Geometry check sheet. Reference: the model listing, model coordinates, mm. A direction names the side the tool comes from. Give positions to 0.01 mm unless a question says otherwise; leave off trailing zeros. Order: outer loops, then holes, each group sorted by start corner. A loop starts at its lowest first (then second) coordinate and runs counter-clockwise, first axis right, second up. Notation, with made-up numbers: (68.25, -13) - (77.25, -13) arc R19 ccw to (77.25, 16) - close; hole circle Ø1 at (48.5, 45.5). An arc over 180 degrees is marked (long way). Put each result on its own line as item: value. Start each with the question number.
```python
from build123d import *

# Parameters (mm, degrees)
SKETCH2_R             = 22.5
BOSS_EXTRUDE2_DEPTH   = 45
M4_TAPPED_HOLE2_D     = 3.3
M4_TAPPED_HOLE2_DEPTH = 10.1
M4_TAPPED_HOLE2_TIP   = 0.991420021
SKETCH6_R             = 12
BOSS_EXTRUDE3_DEPTH   = 2
SKETCH7_R             = 5
BOSS_EXTRUDE4_DEPTH   = 25
CUT_EXTRUDE1_START    = -20
CUT_EXTRUDE1_DEPTH    = 20
SKETCH9_R             = 21
BOSS_EXTRUDE5_DEPTH   = 70
SKETCH10_R            = 18.5
BOSS_EXTRUDE6_DEPTH   = 3
SKETCH11_R            = 19.5
BOSS_EXTRUDE7_DEPTH   = 1
SKETCH12_R            = 18.5
BOSS_EXTRUDE8_DEPTH   = 7
SKETCH13_W            = 5
SKETCH13_H            = 1.5
BOSS_EXTRUDE9_DEPTH   = 7
SKETCH14_R            = 1.25
CUT_EXTRUDE2_DEPTH    = 100.047968177
FILLET1_R             = 1
FILLET2_R             = 0.5
FILLET3_R             = 0.5


with BuildPart() as part:
    # Sketch2 → Boss-Extrude2 (new body)
    with BuildSketch(Plane.XY):
        with Locations(Location((0, 0, 0), (0, 0, 180))):
            Circle(SKETCH2_R)
    extrude(amount=BOSS_EXTRUDE2_DEPTH)

    # M4 Tapped Hole2
    with Locations(Plane(origin=(0, 17, 45), x_dir=(1, 0, 0), z_dir=(0, 0, 1))):
        with Locations((0, 0), (17, -17), (0, -34), (-17, -17)):
            Hole(M4_TAPPED_HOLE2_D / 2, depth=M4_TAPPED_HOLE2_DEPTH)
            with Locations((0, 0, -(M4_TAPPED_HOLE2_DEPTH + M4_TAPPED_HOLE2_TIP / 2))):  # 118° drill point
                Cone(0, M4_TAPPED_HOLE2_D / 2, M4_TAPPED_HOLE2_TIP, mode=Mode.SUBTRACT)

    # Sketch6 → Boss-Extrude3 (add)
    with BuildSketch(Plane.XY.offset(45)):
        Circle(SKETCH6_R)
    extrude(amount=BOSS_EXTRUDE3_DEPTH)

    # Sketch7 → Boss-Extrude4 (add)
    with BuildSketch(Plane.XY.offset(47)):
        Circle(SKETCH7_R)
    extrude(amount=BOSS_EXTRUDE4_DEPTH)

    # Sketch8 → Cut-Extrude1 (cut)
    with BuildSketch(Plane.XY.offset(72).offset(CUT_EXTRUDE1_START)):
        with BuildLine():
            Line((-3.570714214, 3.5), (3.570714214, 3.5))
            ThreePointArc((3.570714214, 3.5), (0, 5), (-3.570714214, 3.5))
        make_face()
    extrude(amount=CUT_EXTRUDE1_DEPTH, mode=Mode.SUBTRACT)

    # Sketch9 → Boss-Extrude5 (add)
    with BuildSketch(Plane(origin=(0, 0, 0), x_dir=(-1, 0, 0), z_dir=(0, 0, -1))):
        Circle(SKETCH9_R)
    extrude(amount=BOSS_EXTRUDE5_DEPTH)

    # Sketch10 → Boss-Extrude6 (add)
    with BuildSketch(Plane(origin=(0, 0, -70), x_dir=(-1, 0, 0), z_dir=(0, 0, -1))):
        Circle(SKETCH10_R)
    extrude(amount=BOSS_EXTRUDE6_DEPTH)

    # Sketch11 → Boss-Extrude7 (add)
    with BuildSketch(Plane(origin=(0, 0, -73), x_dir=(-1, 0, 0), z_dir=(0, 0, -1))):
        Circle(SKETCH11_R)
    extrude(amount=BOSS_EXTRUDE7_DEPTH)

    # Sketch12 → Boss-Extrude8 (add)
    with BuildSketch(Plane(origin=(0, 0, -74), x_dir=(-1, 0, 0), z_dir=(0, 0, -1))):
        Circle(SKETCH12_R)
    extrude(amount=BOSS_EXTRUDE8_DEPTH)

    # Sketch13 → Boss-Extrude9 (add)
    with BuildSketch(Plane(origin=(0, 0, -81), x_dir=(-1, 0, 0), z_dir=(0, 0, -1))):
        with Locations((0, -16.25)):
            Rectangle(SKETCH13_W, SKETCH13_H)
        with Locations((0, 16.25)):
            Rectangle(SKETCH13_W, SKETCH13_H)
    extrude(amount=BOSS_EXTRUDE9_DEPTH)

    # Sketch14 → Cut-Extrude2 (cut, through all)
    with BuildSketch(Plane.XZ.offset(17)):
        with Locations(Location((0, -86.5, 0), (0, 0, 270))):
            Circle(SKETCH14_R)
    extrude(amount=-CUT_EXTRUDE2_DEPTH, mode=Mode.SUBTRACT)

    # Fillet1
    fillet1_edges = [part.edges().sort_by_distance(p)[0] for p in [
        (2.5, 16.25, -88),
        (-2.5, 16.25, -88),
        (-2.5, -16.25, -88),
        (2.5, -16.25, -88),
    ]]
    fillet(fillet1_edges, radius=FILLET1_R)

    # Fillet2
    fillet2_edges = [part.edges().sort_by_distance(p)[0] for p in [
        (18.5, 0, -81),
    ]]
    fillet(fillet2_edges, radius=FILLET2_R)

    # Fillet3
    fillet3_edges = [part.edges().sort_by_distance(p)[0] for p in [
        (22.5, 0, 0),
    ]]
    fillet(fillet3_edges, radius=FILLET3_R)


solid = part.part
```
Item 1: Gauge pin test, flat ends, axial feed: pin 1 Ø3 at (x, y) = (6.5, 1) entering from +Z; pin 2 Ø1.2 at (x, y) = (-2, 4.5) entering from +Z; pin 3 Ø1.5 at (x, z) = (-1, -83.5) entering from -Y; pin 4 Ø3 at (y, z) = (5.5, 53.5) entering from -X. Record the tip position at first contact, or that the pin passes through.
Item 2: Cross-section at C-C (z = -26.5). Enter the section's corners in (x, y), and give its area (3 significant figures).
Item 3: Cross-section at A-A (z = 29). Enter the section's corners in (x, y), and give its area (3 significant figures).
Item 4: Set-up check for faces 5 (the face through (-20.03, 6.31, -34.51)), 6 (the face through (0, -19, -70)), 7 (the face through (0, -15.5, -84)), 8 (the face through (-18.574, 0.496, 39.879)): record each of +Z, -Z, +X, -X, +Y, -Y from which the full face is reachable in a straight line by a thin tool's end or side.
Item 5: Thickness scan on line 1 along Y through (x, z) = (0, 42); line 2 along X through (y, z) = (1, -51); line 3 along Z through (x, y) = (11, -11). Record the ranges inside material, lowest first.
Item 6: Release check for a two-part mould opening along Y. For faces 1 (the face through (15.476, -0.632, 39.879)), 2 (the face through (0, 15.5, -84)), 3 (the face through (-10.382, 19.961, 22.438)), 4 (the face through (-10, 10, 45)) record: +Y half, -Y half, draft (parallel to the pull), parting line (faces both ways), or undercut.
Item 7: Cross-section at B-B (z = 57). Enter the section's corners in (x, y), and give its area (3 significant figures).
Recorded:
1. pin 1: stops at z = 47
1. pin 2: stops at z = 52
1. pin 3: stops at y = -17
1. pin 4: passes through
2. outline: circle Ø42 at (0, 0)
2. area: 1,390 mm^2
3. outline: circle Ø45 at (0, 0)
3. area: 1,590 mm^2
4. face 5: -Z
4. face 6: none
4. face 7: -Z, +X, -X
4. face 8: +Z
5. line 1: y = -22.5 to -18.65, -15.35 to 15.35, 18.65 to 22.5
5. line 2: x = -20.98 to 20.98
5. line 3: z = -81 to 45
6. face 1: undercut
6. face 2: undercut
6. face 3: parting line
6. face 4: draft
7. outline: (-3.57, 3.5) arc R5 ccw (long way) to (3.57, 3.5) - close
7. area: 71.2 mm^2
